Here's how the part is built. I have some questions about the finished solid (model axes, mm). Face numbers are marked on the shaded views. A direction names the side the tool comes from. Coordinates: 2 decimals unless noted, no trailing zeros. Write each loop counter-clockwise with the first axis right and the second up, starting at its lowest first coordinate (ties: lowest second). Pieces come first, ordered by that corner, then holes. Notation, with made-up numbers: (-13, 39) -> (27, 39) arc R4 cw to (27, 43) -> close; hole circle Ø6 at (-20.5, 22). An arc over 180 degrees is marked (long way). Answer in a Markdown table with one row per item. Add a question column.
from build123d import *

# Parameters (mm, degrees)
F1_DEPTH = 38.1
F3_DEPTH = 152.4
F5_W     = 203.2
F5_H     = 254
F6_DEPTH = 254
F7_R     = 12.7
F8_DEPTH = 25.4


with BuildPart() as f1:
    # F0 (on Right) → F1 (new body, symmetric)
    with BuildSketch(Plane.YZ):
        with BuildLine():
            ThreePointArc((33.242401, 703.56663), (75.487635, 624.604952), (13.472578, 560.000469))
            Line((13.472578, 560.000469), (-558.8, 457.2))
            Line((-558.8, 457.2), (-914.4, 457.2))
            Line((-914.4, 457.2), (-914.4, 0))
            Line((-914.4, 0), (762, 0))
            Line((762, 0), (762, 1752.6))
            Line((762, 1752.6), (0, 1752.6))
            Line((0, 1752.6), (-558.8, 1295.4))
            Line((-558.8, 1295.4), (-914.4, 1295.4))
            Line((-914.4, 1295.4), (-914.4, 990.6))
            Line((-914.4, 990.6), (-558.8, 990.6))
            Line((-558.8, 990.6), (33.242401, 703.56663))
        make_face()
    extrude(amount=F1_DEPTH, both=True)


with BuildPart() as f3:
    # F2 (on Right) → F3 (new body, symmetric)
    with BuildSketch(Plane.YZ):
        with BuildLine():
            Line((-558.8, 990.6), (33.242401, 703.56663))
            ThreePointArc((33.242401, 703.56663), (75.487635, 624.604952), (13.472578, 560.000469))
            Line((13.472578, 560.000469), (-558.8, 457.2))
            Line((-558.8, 457.2), (-914.4, 457.2))
            Line((-914.4, 457.2), (-914.4, 0))
            Line((-914.4, 0), (762, 0))
            Line((762, 0), (762, 1752.6))
            Line((762, 1752.6), (0, 1752.6))
            Line((0, 1752.6), (-558.8, 1295.4))
            Line((-558.8, 1295.4), (-914.4, 1295.4))
            Line((-914.4, 1295.4), (-914.4, 990.6))
            Line((-914.4, 990.6), (-558.8, 990.6))
        make_face()
        with BuildLine():
            Line((698.5, 1689.1), (698.5, 63.5))
            Line((698.5, 63.5), (-850.9, 63.5))
            Line((-850.9, 63.5), (-850.9, 393.7))
            Line((-850.9, 393.7), (-553.141856, 393.7))
            Line((-553.141856, 393.7), (24.699726, 497.50086))
            ThreePointArc((24.699726, 497.50086), (138.393997, 615.942412), (60.944402, 760.705489))
            Line((60.944402, 760.705489), (-544.218653, 1054.1))
            Line((-544.218653, 1054.1), (-850.9, 1054.1))
            Line((-850.9, 1054.1), (-850.9, 1231.9))
            Line((-850.9, 1231.9), (-536.132825, 1231.9))
            Line((-536.132825, 1231.9), (22.667175, 1689.1))
            Line((22.667175, 1689.1), (698.5, 1689.1))
        make_face(mode=Mode.SUBTRACT)
    extrude(amount=F3_DEPTH, both=True)


with BuildPart() as f1_1:
    add(f1.part)

    # F4: union F3
    add(f3.part)

    # F5 (on face) → F6 (join)
    with BuildSketch(Plane(origin=(0, 0, 990.6), x_dir=(1, 0, 0), z_dir=(0, 0, -1))):
        with Locations((0, 736.6)):
            Rectangle(F5_W, F5_H)
    extrude(amount=F6_DEPTH)

    # F7 (on face) → F8 (join)
    with BuildSketch(Plane(origin=(0, 0, 736.6), x_dir=(1, 0, 0), z_dir=(0, 0, -1))):
        with Locations((0, 736.6)):
            Circle(F7_R)
    extrude(amount=F8_DEPTH)


solid = f1_1.part
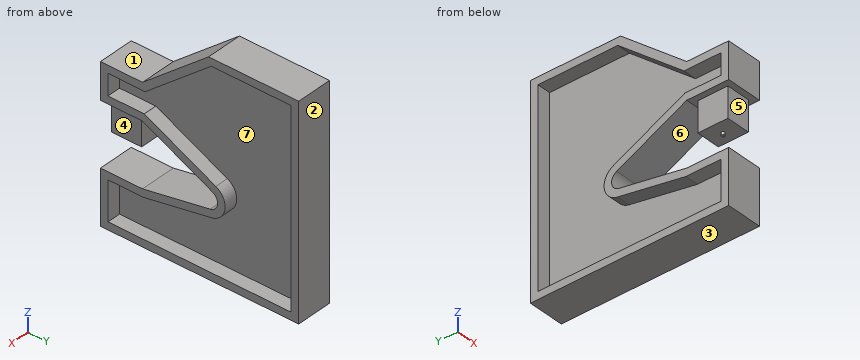
Q1. I'm going to push flat-ended pins straight in: P1, Ø10, axis at x = -3.5, y = -480.5, coming from the +Z side; P2, Ø5, axis at x = -44.5, y = -433, coming from the +Z side; P3, Ø1.5, axis at y = -625, z = 340.5, coming from the +X side. Where does each tip first touch, or does it pass through?
Q2. Imagine slicing it at A-A on x = 65. Please give me the cut outline in (y, z).
Q3. Imagine slicing it at D-D on z = 268. Please give me the cut outline in (x, y).
Q4. For the marked faces 5, 6 and 7, which set-ups out of +Z, -Z, +X, -X, +Y, -Y let a thin tool reach every point of the face, with its end or its side?
Q5. Imagine slicing it at C-C on y = -115. Please give me the cut outline in (x, z).
Q6. I need wall thicknesses on line 1 (Z direction, x = -70, y = -731); line 2 (Z direction, x = 83.5, y = -559.5); line 3 (Y direction, x = 80.5, z = 932). Which ranges of each line are inside material? Lowest first, please. Write a range as [from, to].
Q7. If we mould it in two halves opening along Z, with no side actions, what happens to the marked faces 1, 2, 3 and 4? For each: pulls with the +Z half, pulls with the -Z half, needs draft (parallel to the pull), parting line crosses it, or undercut.
Q8. Imagine slicing it at B-B on z = 958. Please give me the cut outline in (x, y), plus the area to 3 significant figures.
Result sheet:
| question | item | result |
|---|---|---|
| 1 | P1 | stops at z = 1363.55 |
| 1 | P2 | stops at z = 1400.37 |
| 1 | P3 | stops at x = 38.1 |
| 2 | outline | (-914.4, 0) -> (762, 0) -> (762, 1752.6) -> (0, 1752.6) -> (-558.8, 1295.4) -> (-914.4, 1295.4) -> (-914.4, 990.6) -> (-863.6, 990.6) -> (-863.6, 736.6) -> (-609.6, 736.6) -> (-609.6, 990.6) -> (-558.8, 990.6) -> (33.24, 703.57) arc R76.2 cw to (13.47, 560) -> (-558.8, 457.2) -> (-914.4, 457.2) -> close; hole (-850.9, 63.5) -> (698.5, 63.5) -> (698.5, 1689.1) -> (22.67, 1689.1) -> (-536.13, 1231.9) -> (-850.9, 1231.9) -> (-850.9, 1054.1) -> (-544.22, 1054.1) -> (60.94, 760.71) arc R139.7 cw to (24.7, 497.5) -> (-553.14, 393.7) -> (-850.9, 393.7) -> close |
| 3 | outline | (-152.4, -914.4) -> (152.4, -914.4) -> (152.4, -850.9) -> (38.1, -850.9) -> (38.1, 698.5) -> (152.4, 698.5) -> (152.4, 762) -> (-152.4, 762) -> (-152.4, 698.5) -> (-38.1, 698.5) -> (-38.1, -850.9) -> (-152.4, -850.9) -> close |
| 4 | face 5 | +X, -X, -Y |
| 4 | face 6 | +X, -X |
| 4 | face 7 | +X |
| 5 | outline | (-152.4, 0) -> (152.4, 0) -> (152.4, 63.5) -> (38.1, 63.5) -> (38.1, 472.41) -> (152.4, 472.41) -> (152.4, 536.92) -> (-152.4, 536.92) -> (-152.4, 472.41) -> (-38.1, 472.41) -> (-38.1, 63.5) -> (-152.4, 63.5) -> close; (-152.4, 775.44) -> (152.4, 775.44) -> (152.4, 846.01) -> (38.1, 846.01) -> (38.1, 1576.46) -> (152.4, 1576.46) -> (152.4, 1658.51) -> (-152.4, 1658.51) -> (-152.4, 1576.46) -> (-38.1, 1576.46) -> (-38.1, 846.01) -> (-152.4, 846.01) -> close |
| 6 | line 1 | z = [0, 63.5], [393.7, 457.2], [736.6, 1054.1], [1231.9, 1295.4] |
| 6 | line 2 | z = [0, 63.5], [393.7, 457.2], [990.6, 1054.1], [1231.9, 1295.4] |
| 6 | line 3 | y = [-863.6, -609.6], [-437.93, -292.37], [698.5, 762] |
| 7 | face 1 | pulls with the +Z half |
| 7 | face 2 | needs draft |
| 7 | face 3 | pulls with the -Z half |
| 7 | face 4 | undercut |
| 8 | outline | (-152.4, -491.56) -> (152.4, -491.56) -> (152.4, -346) -> (38.1, -346) -> (38.1, 698.5) -> (152.4, 698.5) -> (152.4, 762) -> (-152.4, 762) -> (-152.4, 698.5) -> (-38.1, 698.5) -> (-38.1, -346) -> (-152.4, -346) -> close; (-101.6, -863.6) -> (101.6, -863.6) -> (101.6, -609.6) -> (-101.6, -609.6) -> close |
| 8 | area | 195,000 mm^2 |
